from build123d import *

# Parameters (mm, degrees)
BOSS_EXTRUDE1_DEPTH = 20
SKETCH2_R           = 1.65
SKETCH2_W           = 6
SKETCH2_H           = 6.9
BOSS_EXTRUDE2_DEPTH = 19
CUT_EXTRUDE1_DEPTH  = 10


with BuildPart() as part:
    # Sketch1 → Boss-Extrude1 (new body)
    with BuildSketch(Plane(origin=(0, 0, 0), x_dir=(1, 0, 0), z_dir=(0, 1, 0))):
        Polygon((-61.870068173, 40.5), (61.870068173, 40.5), (73.25, 28.287390235), (73.25, -28.33163873), (26.325219162, -75), (-26.325219162, -75), (-73.25, -28.33163873), (-73.25, 28.287390235), align=None)
        Polygon((-61, 38.5), (61, 38.5), (71.25, 27.5), (71.25, -27.5), (25.5, -73), (-25.5, -73), (-71.25, -27.5), (-71.25, 27.5), align=None, mode=Mode.SUBTRACT)
    extrude(amount=BOSS_EXTRUDE1_DEPTH)

    # Sketch2 → Boss-Extrude2 (add)
    # profile 1 of 6: a face of its own
    with BuildSketch(Plane(origin=(0, 0, 0), x_dir=(1, 0, 0), z_dir=(0, 1, 0))):
        Polygon((-40.880359301, -57.703686378), (-35.861623629, -52.657375236), (-31.607375236, -56.888376371), (-36.626110907, -61.934687513), align=None)
        with Locations(Location((-35.85, -56.9, 0), (0, 0, 270))):
            Circle(SKETCH2_R, mode=Mode.SUBTRACT)
    # profile 2 of 6: a face of its own
    with BuildSketch(Plane(origin=(0, 0, 0), x_dir=(1, 0, 0), z_dir=(0, 1, 0))):
        Polygon((-60.73445685, -37.958081166), (-55.661623629, -32.857375236), (-51.407375236, -37.088376371), (-56.480208456, -42.189082301), align=None)
        with Locations(Location((-55.65, -37.1, 0), (0, 0, 270))):
            Circle(SKETCH2_R, mode=Mode.SUBTRACT)
    # profile 3 of 6: a face of its own
    with BuildSketch(Plane(origin=(0, 0, 0), x_dir=(1, 0, 0), z_dir=(0, 1, 0))):
        with Locations((-55.65, 35.05)):
            Rectangle(SKETCH2_W, SKETCH2_H)
        with Locations(Location((-55.65, 34.6, 0), (0, 0, 270))):
            Circle(SKETCH2_R, mode=Mode.SUBTRACT)
    # profile 4 of 6: a face of its own
    with BuildSketch(Plane(origin=(0, 0, 0), x_dir=(1, 0, 0), z_dir=(0, 1, 0))):
        with Locations((55.65, 35.05)):
            Rectangle(SKETCH2_W, SKETCH2_H)
        with Locations(Location((55.65, 34.6, 0), (0, 0, 90))):
            Circle(SKETCH2_R, mode=Mode.SUBTRACT)
    # profile 5 of 6: a face of its own
    with BuildSketch(Plane(origin=(0, 0, 0), x_dir=(1, 0, 0), z_dir=(0, 1, 0))):
        Polygon((56.480208456, -42.189082301), (60.73445685, -37.958081166), (55.661623629, -32.857375236), (51.407375236, -37.088376371), align=None)
        with Locations(Location((55.65, -37.1, 0), (0, 0, 90))):
            Circle(SKETCH2_R, mode=Mode.SUBTRACT)
    # profile 6 of 6: a face of its own
    with BuildSketch(Plane(origin=(0, 0, 0), x_dir=(1, 0, 0), z_dir=(0, 1, 0))):
        Polygon((36.626110907, -61.934687513), (40.880359301, -57.703686378), (35.861623629, -52.657375236), (31.607375236, -56.888376371), align=None)
        with Locations(Location((35.85, -56.9, 0), (0, 0, 90))):
            Circle(SKETCH2_R, mode=Mode.SUBTRACT)
    extrude(amount=BOSS_EXTRUDE2_DEPTH)

    # Sketch3 → Cut-Extrude1 (cut)
    with BuildSketch(Plane.ZY.offset(73.25)):
        with BuildLine():
            Line((28.33163873, 0), (13.33163873, 0))
            Line((13.33163873, 0), (13.33163873, 6))
            ThreePointArc((13.33163873, 6), (14.503211605, 8.828427125), (17.33163873, 10))
            Line((17.33163873, 10), (24.33163873, 10))
            ThreePointArc((24.33163873, 10), (27.160065854, 8.828427125), (28.33163873, 6))
            Line((28.33163873, 6), (28.33163873, 0))
        make_face()
    extrude(amount=-CUT_EXTRUDE1_DEPTH, mode=Mode.SUBTRACT)


solid = part.part
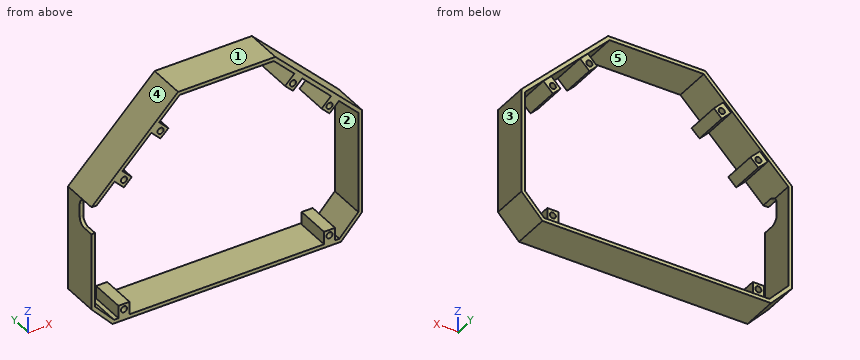
Verification items for the finished model (mm, model axes). Face numbers are marked on the shaded views. A direction names the side the tool comes from. Coordinates: 2 decimals unless noted, no trailing zeros. Write each loop counter-clockwise with the first axis right and the second up, starting at its lowest first coordinate (ties: lowest second). Pieces come first, ordered by that corner, then holes. Notation, with made-up numbers: (25, 22) - (48, 22) arc R19 ccw to (48, 57) - close; hole circle Ø6 at (71, 85.5). An arc over 180 degrees is marked (long way). Answer as a JSON object with one key per item and string values.
(1) Cross-section at C-C on x = 46. Record the cut outline in (y, z), plus the area to 3 significant figures.
Report:
{"outline": "(0, -40.5) - (20, -40.5) - (20, -38.5) - (0, -38.5) - close; (0, 52.61) - (20, 52.61) - (20, 55.43) - (0, 55.43) - close", "area": "96.4 mm^2"}
(2) Cross-section at B-B on z = -34.6. Record the cut outline in (x, y), plus the area to 3 significant figures.
Report:
{"outline": "(-67.37, 0) - (-64.63, 0) - (-64.63, 20) - (-67.37, 20) - close; (-58.65, 0) - (-57.3, 0) - (-57.3, 19) - (-58.65, 19) - close; (-54, 0) - (-52.65, 0) - (-52.65, 19) - (-54, 19) - close; (52.65, 0) - (54, 0) - (54, 19) - (52.65, 19) - close; (57.3, 0) - (58.65, 0) - (58.65, 19) - (57.3, 19) - close; (64.63, 0) - (67.37, 0) - (67.37, 20) - (64.63, 20) - close", "area": "212 mm^2"}
(3) Cross-section at A-A on z = 65. Record the cut outline in (x, y).
Report:
{"outline": "(-36.38, 0) - (-33.54, 0) - (-33.54, 20) - (-36.38, 20) - close; (33.54, 0) - (36.38, 0) - (36.38, 20) - (33.54, 20) - close"}
(4) Tool access check on the marked faces 4 and 5. Record the directions out of +Z, -Z, +X, -X, +Y, -Y that give a thin tool (end or side, any length) a straight path to the whole face; none if there is none.
Report:
{"face 4": "+Z, -X, +Y, -Y", "face 5": "+Y, -Y"}
(5) Mould release check, pull along Z, two halves, no side actions. Record for the marked faces 1, 2 and 3: pulls with the +Z half, pulls with the -Z half, needs draft (parallel to the pull), parting line crosses it, or undercut.
Report:
{"face 1": "pulls with the +Z half", "face 2": "undercut", "face 3": "needs draft"}
(6) Thickness scan on line 1 along X through (y, z) = (17, -23.5); line 2 along X through (y, z) = (5, -34.6); line 3 along X through (y, z) = (8.5, 37.1). Record the ranges inside material, lowest first.
Report:
{"line 1": "-73.25 to -71.25, 71.25 to 73.25", "line 2": "-67.37 to -64.63, -58.65 to -57.3, -54 to -52.65, 52.65 to 54, 57.3 to 58.65, 64.63 to 67.37", "line 3": "-64.43 to -61.6, -59.88 to -57.3, -54 to -51.42, 51.42 to 54, 57.3 to 59.88, 61.6 to 64.43"}
(7) Gauge pin test, flat ends, axial feed: pin 1 Ø6.5 at (x, y) = (55, 7) entering from +Z; pin 2 Ø1.6 at (x, z) = (-72, 20) entering from -Y; pin 3 Ø1.8 at (x, z) = (-57, -36.5) entering from +Y; pin 4 Ø3 at (x, z) = (55.65, 37.1) entering from -Y. Record the tip position at first contact, or that the pin passes through.
Report:
{"pin 1": "z = 49.71", "pin 2": "y = 10", "pin 3": "y = 19", "pin 4": "through"}
(8) Cross-section at D-D on y = 4.25. Give the number of separate pieces and of enclosed holes in the cut face, plus the area to 3 significant figures.
Report:
{"separate pieces": "1", "enclosed holes": "6", "area": "1,070 mm^2"}
